Verification items for the finished model (mm, model axes). Give positions to 0.01 mm unless a question says otherwise; leave off trailing zeros. Order: outer loops, then holes, each group sorted by start corner. A loop starts at its lowest first (then second) coordinate and runs counter-clockwise, first axis right, second up.
from build123d import *

# Parameters (mm, degrees)
SKETCH1_W           = 35
SKETCH1_H           = 45
BOSS_EXTRUDE1_DEPTH = 12
SKETCH2_R           = 10
CUT_EXTRUDE1_DEPTH  = 59.258046655
SKETCH3_R           = 1.75
CUT_EXTRUDE2_DEPTH  = 25


with BuildPart() as part:
    # Sketch1 → Boss-Extrude1 (new body)
    with BuildSketch(Plane(origin=(0, 0, 0), x_dir=(1, 0, 0), z_dir=(0, 1, 0))):
        with Locations((17.5, 22.5)):
            Rectangle(SKETCH1_W, SKETCH1_H)
    extrude(amount=BOSS_EXTRUDE1_DEPTH)

    # Sketch2 → Cut-Extrude1 (cut, through all)
    with BuildSketch(Plane.XY):
        with Locations((17.5, 12)):
            Circle(SKETCH2_R)
    extrude(amount=-CUT_EXTRUDE1_DEPTH, mode=Mode.SUBTRACT)

    # Sketch3 → Cut-Extrude2 (cut)
    with BuildSketch(Plane(origin=(0, 12, 0), x_dir=(1, 0, 0), z_dir=(0, 1, 0))):
        with Locations(Location((30.9, 22.5, 0), (0, 0, 270))):
            Circle(SKETCH3_R)
        with Locations(Location((4.1, 22.5, 0), (0, 0, 270))):
            Circle(SKETCH3_R)
    extrude(amount=-CUT_EXTRUDE2_DEPTH, mode=Mode.SUBTRACT)


solid = part.part
(1) Section check A-A, the plane x = 30.9. Enter the section's corners in (y, z).
Solved:
outline: (0, -45) - (12, -45) - (12, -24.25) - (0, -24.25) - close; (0, -20.75) - (12, -20.75) - (12, 0) - (0, 0) - close
(2) Section check D-D, the plane x = 17.5. Enter the section's corners in (y, z), then the cut area to 3 significant figures.
Solved:
outline: (0, -45) - (2, -45) - (2, 0) - (0, 0) - close
area: 90.0 mm2
(3) Section check C-C, the plane z = -4. Enter the section's corners in (x, y), then the cut area to 3 significant figures.
Solved:
outline: (0, 0) - (35, 0) - (35, 12) - (27.5, 12) arc R10 cw to (7.5, 12) - (0, 12) - close
area: 263 mm2
(4) Go/stop test with flat-tipped pins: pin 1 (3 mm diameter, centred on x = 4.1, z = -22.5, fed in from -Y); pin 2 (4 mm diameter, centred on x = 14, z = -10, fed in from +Y). Record where each tip stops, or that it passes through.
Solved:
pin 1: passes through
pin 2: stops at y = 3.65
(5) Release check for a two-part mould opening along Z. For faces 1 (the flat face through (17, 1, -45)), 2 (the cylindrical face through (30.98, 6.08, -24.25)), 3 (the cylindrical face through (17.3, 2, -22.2)) record: pulls with the +Z half, pulls with the -Z half, needs draft (parallel to the pull), parting line crosses it, or undercut.
Solved:
face 1: pulls with the -Z half
face 2: undercut
face 3: needs draft
(6) Scan lines: line 1 (X direction, y = 2.75, z = -22.5); line 2 (X direction, y = 7.5, z = -22.5); line 3 (X direction, y = 6, z = -9). Record each from-to range of solid material in increasing order.
Solved:
line 1: x = 0 to 2.35, 5.85 to 13.7, 21.3 to 29.15, 32.65 to 35
line 2: x = 0 to 2.35, 5.85 to 8.57, 26.43 to 29.15, 32.65 to 35
line 3: x = 0 to 9.5, 25.5 to 35
(7) Section check B-B, the plane y = 3. Enter the section's corners in (x, z), then the cut area to 3 significant figures.
Solved:
outline: (0, -45) - (13.14, -45) - (13.14, 0) - (0, 0) - close; (21.86, -45) - (35, -45) - (35, 0) - (21.86, 0) - close; hole circle Ø3.5 at (4.1, -22.5); hole circle Ø3.5 at (30.9, -22.5)
area: 1,160 mm2
